Can you work these out from the drawing? Everything is in mm from the part's minimum corner. Round coordinates to 2 decimals unless told otherwise and drop trailing zeros. Loops run counter-clockwise (first coordinate to the right, second up) from the corner with the lowest first, then second, coordinate; pieces in that order, holes last. Notation, with made-up numbers: (-27, 71.5) -> (-12, 71.5) arc R25 ccw to (-12, 107.5) -> close; hole circle Ø2 at (-11, 59). An arc over 180 degrees is marked (long way). Answer as a JSON object with one key per item and string values.
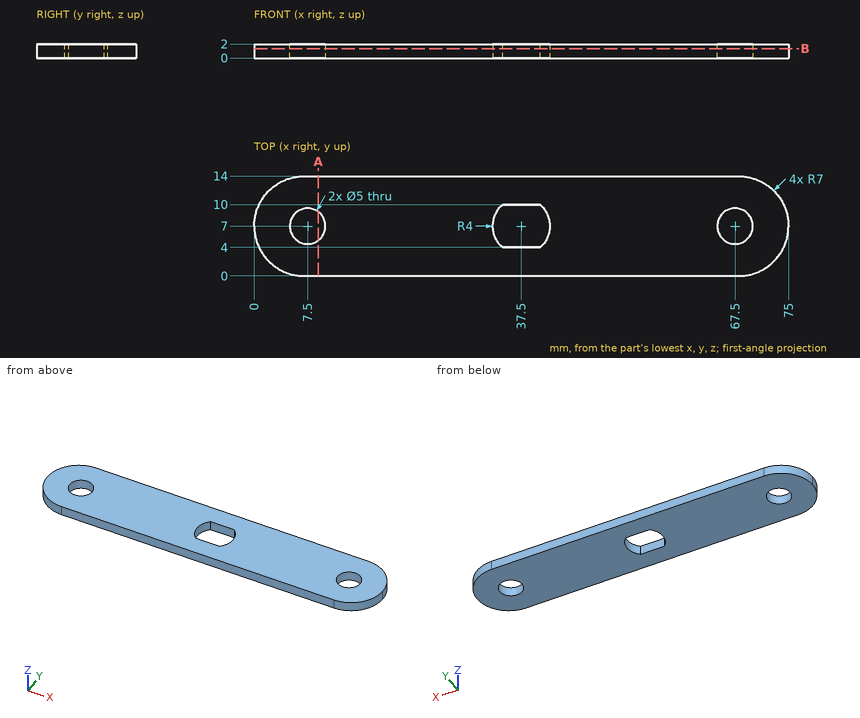
Q1. I want a section at B-B, the plane z = 1.35. Give the number of separate pieces and of enclosed holes in the cut face, then the cut area to 3 significant figures.
Determined:
{"separate pieces": "1", "enclosed holes": "3", "area": "926 mm²"}
Q2. I'm going to push a flat-ended pin straight in: pin 1 (4 mm diameter, centred on x = 7.5, y = 7, fed in from +Z). Where does the tip first touch, or does it pass through?
Determined:
{"pin 1": "through"}
Q3. I want a section at A-A, the plane x = 9. Write out the boundary of the cut face in (y, z).
Determined:
{"outline": "(0, 0) -> (5, 0) -> (5, 2) -> (0, 2) -> close; (9, 0) -> (14, 0) -> (14, 2) -> (9, 2) -> close"}
Q4. If I drill on L1, parallel to X at y = 6.75, z = 0.2; L2, parallel to Y at x = 67.5, z = 1.15; L3, parallel to Y at x = 37, z = 0.25, over which ranges is the centre line in solid material (lowest first)? Write a range as [from, to].
Determined:
{"L1": "[0, 5.01], [9.99, 33.51], [41.49, 65.01], [69.99, 75]", "L2": "[0, 4.5], [9.5, 14]", "L3": "[0, 4], [10, 14]"}
